Verification items for the finished model (mm, model axes). A direction names the side the tool comes from. Coordinates: 2 decimals unless noted, no trailing zeros. Order: outer loops, then holes, each group sorted by start corner. A loop starts at its lowest first (then second) coordinate and runs counter-clockwise, first axis right, second up. Notation, with made-up numbers: (21, 38.5) -> (39, 38.5) arc R9 cw to (39, 52.5) -> close; hole circle Ø8 at (53.5, 52). An arc over 180 degrees is marked (long way). Write each question's results on one line, items separated by ' | '. Start each with the question number.
(1) Thickness scan on probe 1 along Y at (x, z) = (111, 20.5); probe 2 along X at (y, z) = (73.5, 23); probe 3 along Y at (x, z) = (177, 40.5). Record the ranges inside material, lowest first. Write a range as [from, to].
(2) Cross-section at C-C on x = 184.5. Enter the section's corners in (y, z).
(3) Cross-section at A-A on z = 57. Enter the section's corners in (x, y), and give its area (3 significant figures).
(4) Draft check along Y on faces 1 (the flat face through (113, 0, 37)), 2 (the flat face through (230, 54, 37)), 3 (the flat face through (113, 110, 37)), 4 (the cylindrical face through (200.63, 24.11, 40.51)). Enter one of: +Y half, -Y half, draft (parallel to the pull), parting line (faces both ways), or undercut.
(5) Set-up check for faces 5 (the flat face through (0, 54, 37)), 6 (the flat face through (111, 79, 6)): record each of +Z, -Z, +X, -X, +Y, -Y from which the full face is reachable in a straight line by a thin tool's end or side.
(6) Cross-section at B-B on y = 31. Enter the section's corners in (x, z), and give its area (3 significant figures).
(7) Go/stop test with a flat-tipped pin: pin 1 (11 mm diameter, centred on x = 109.5, y = 75.5, fed in from +Z). Record where the tip stops, or that it passes through.
(8) Cross-section at D-D on x = 111. Enter the section's corners in (y, z), and give its area (3 significant figures).
```python
from build123d import *

# Parameters (mm, degrees)
CYLINDER001_R     = 18
CYLINDER001_DEPTH = 70
CYLINDER_R        = 18
CYLINDER_DEPTH    = 70
CYLINDER005_R     = 18
CYLINDER005_DEPTH = 70
CYLINDER004_R     = 18
CYLINDER004_DEPTH = 70
CYLINDER003_R     = 18
CYLINDER003_DEPTH = 70
CYLINDER002_R     = 18
CYLINDER002_DEPTH = 70
BOX_W             = 230
BOX_H             = 110
BOX_DEPTH         = 76


with BuildPart() as cylinder001:
    # Cylinder001 → Cylinder001 (new body)
    with BuildSketch(Plane(origin=(39, 79, 6), x_dir=(1, 0, 0), z_dir=(0, 0, 1))):
        Circle(CYLINDER001_R)
    extrude(amount=CYLINDER001_DEPTH)


with BuildPart() as fusion:
    # Cylinder → Cylinder (new body)
    with BuildSketch(Plane(origin=(39, 31, 6), x_dir=(1, 0, 0), z_dir=(0, 0, 1))):
        Circle(CYLINDER_R)
    extrude(amount=CYLINDER_DEPTH)

    # Fusion: union Cylinder001
    add(cylinder001.part)


with BuildPart() as cylinder005:
    # Cylinder005 → Cylinder005 (new body)
    with BuildSketch(Plane(origin=(39, 79, 6), x_dir=(1, 0, 0), z_dir=(0, 0, 1))):
        Circle(CYLINDER005_R)
    extrude(amount=CYLINDER005_DEPTH)


with BuildPart() as fusion002:
    # Cylinder004 → Cylinder004 (new body)
    with BuildSketch(Plane(origin=(39, 31, 6), x_dir=(1, 0, 0), z_dir=(0, 0, 1))):
        Circle(CYLINDER004_R)
    extrude(amount=CYLINDER004_DEPTH)

    # Fusion002: union Cylinder005
    add(cylinder005.part)


with BuildPart() as fusion002_1:
    # Fusion002 placement: moved
    add(fusion002.part.moved(Location((145, 0, 0))))


with BuildPart() as cylinder003:
    # Cylinder003 → Cylinder003 (new body)
    with BuildSketch(Plane(origin=(39, 79, 6), x_dir=(1, 0, 0), z_dir=(0, 0, 1))):
        Circle(CYLINDER003_R)
    extrude(amount=CYLINDER003_DEPTH)


with BuildPart() as fusion003:
    # Cylinder002 → Cylinder002 (new body)
    with BuildSketch(Plane(origin=(39, 31, 6), x_dir=(1, 0, 0), z_dir=(0, 0, 1))):
        Circle(CYLINDER002_R)
    extrude(amount=CYLINDER002_DEPTH)

    # Fusion001: union Cylinder003
    add(cylinder003.part)


with BuildPart() as fusion003_1:
    # Fusion001 placement: moved
    add(fusion003.part.moved(Location((72, 0, 0))))

    # Fusion003: union Fusion, Fusion002
    add(fusion.part)
    add(fusion002_1.part)


with BuildPart() as cut:
    # Box → Box (new body)
    with BuildSketch(Plane.XY):
        with Locations((115, 55)):
            Rectangle(BOX_W, BOX_H)
    extrude(amount=BOX_DEPTH)

    # Cut: cut Fusion003
    add(fusion003_1.part, mode=Mode.SUBTRACT)


solid = cut.part
```
Results are:
1) probe 1: y = [0, 13], [49, 61], [97, 110] | probe 2: x = [0, 21.86], [56.14, 93.86], [128.14, 166.86], [201.14, 230] | probe 3: y = [0, 14.42], [47.58, 62.42], [95.58, 110]
2) outline: (0, 0) -> (110, 0) -> (110, 76) -> (96.99, 76) -> (96.99, 6) -> (61.01, 6) -> (61.01, 76) -> (48.99, 76) -> (48.99, 6) -> (13.01, 6) -> (13.01, 76) -> (0, 76) -> close
3) outline: (0, 0) -> (230, 0) -> (230, 110) -> (0, 110) -> close; hole circle Ø36 at (39, 31); hole circle Ø36 at (39, 79); hole circle Ø36 at (111, 31); hole circle Ø36 at (111, 79); hole circle Ø36 at (184, 31); hole circle Ø36 at (184, 79) | area: 19,200 mm2
4) face 1: -Y half | face 2: draft | face 3: +Y half | face 4: undercut
5) face 5: +Z, -Z, -X, +Y, -Y | face 6: +Z
6) outline: (0, 0) -> (230, 0) -> (230, 76) -> (202, 76) -> (202, 6) -> (166, 6) -> (166, 76) -> (129, 76) -> (129, 6) -> (93, 6) -> (93, 76) -> (57, 76) -> (57, 6) -> (21, 6) -> (21, 76) -> (0, 76) -> close | area: 9,920 mm2
7) pin 1: stops at z = 6
8) outline: (0, 0) -> (110, 0) -> (110, 76) -> (97, 76) -> (97, 6) -> (61, 6) -> (61, 76) -> (49, 76) -> (49, 6) -> (13, 6) -> (13, 76) -> (0, 76) -> close | area: 3,320 mm2
